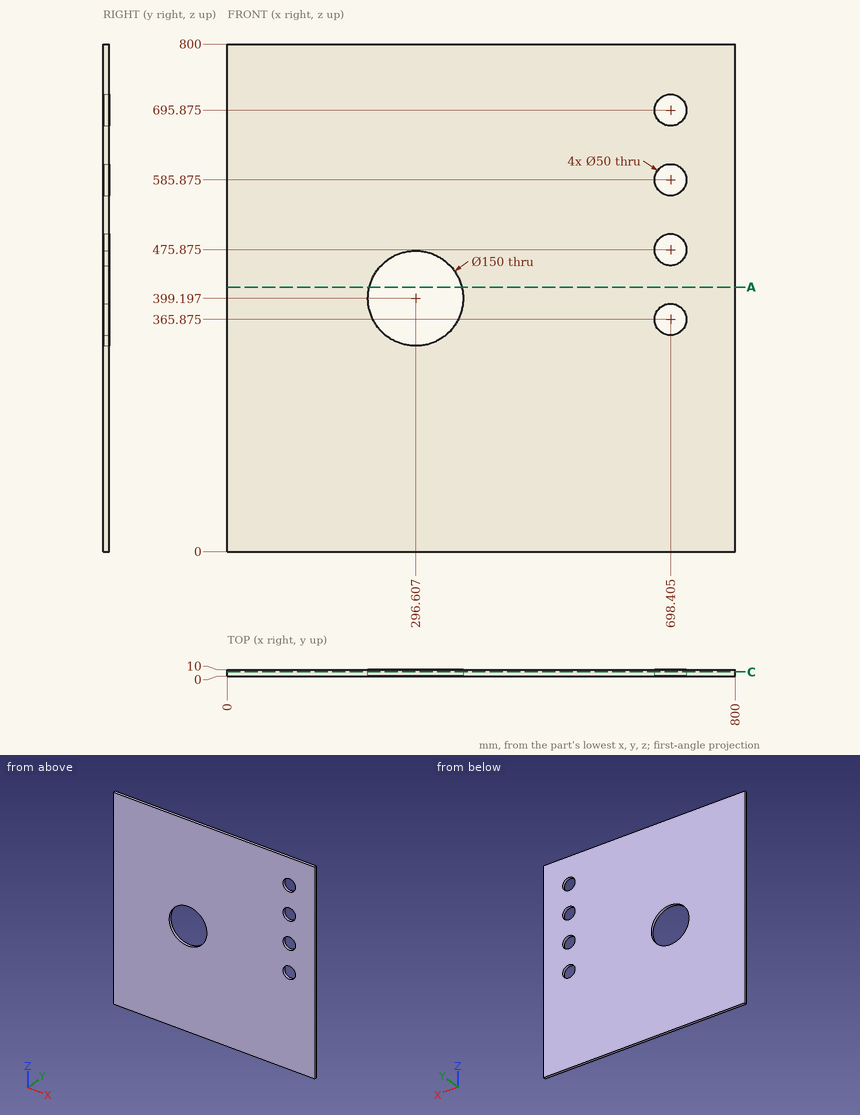
Print and shaded views of the part. All mm, measured from the part's lowest x, y and z. Coordinates: 2 decimals unless noted, no trailing zeros. Order: outer loops, then holes, each group sorted by start corner. A loop starts at its lowest first (then second) coordinate and runs counter-clockwise, first axis right, second up.
(1) Probe L1, parallel to Z at x = 696, y = 6.25; L2, parallel to Z at x = 298, y = 5.5; L3, parallel to X at y = 4.5, z = 401.5. List the from-to ranges inside material, lowest first.
Check sheet entries:
L1: z = 0 to 340.99, 390.76 to 450.99, 500.76 to 560.99, 610.76 to 670.99, 720.76 to 800
L2: z = 0 to 324.21, 474.18 to 800
L3: x = 0 to 221.64, 371.57 to 800
(2) Slice it at C-C, the plane y = 6.5. Write the cut outline in (x, z) (1 decimal).
Check sheet entries:
outline: (0, 0) - (800, 0) - (800, 800) - (0, 800) - close; hole circle Ø150 at (296.6, 399.2); hole circle Ø50 at (698.4, 365.9); hole circle Ø50 at (698.4, 475.9); hole circle Ø50 at (698.4, 585.9); hole circle Ø50 at (698.4, 695.9)
(3) Slice it at A-A, the plane z = 417. Write the cut outline in (x, y), and give its area (3 significant figures).
Check sheet entries:
outline: (0, 0) - (223.75, 0) - (223.75, 10) - (0, 10) - close; (369.46, 0) - (800, 0) - (800, 10) - (369.46, 10) - close
area: 6,540 mm2
